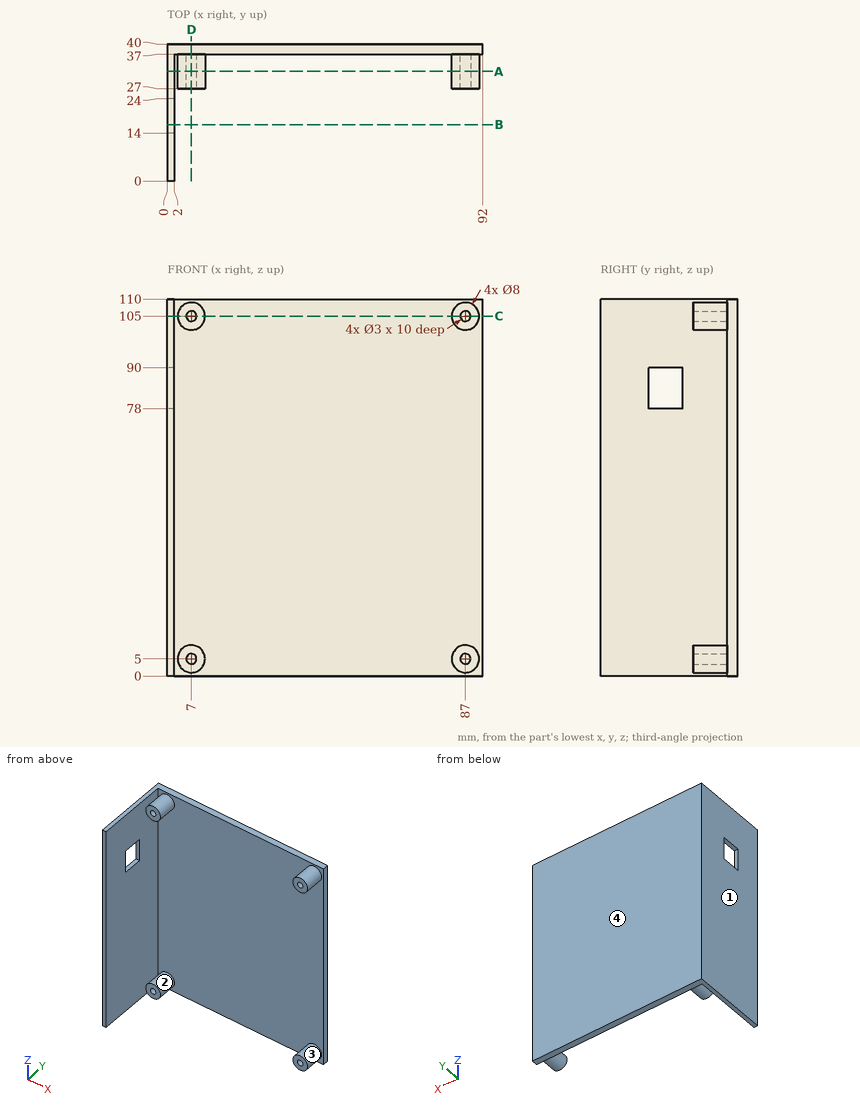
The figure shows three views and two pictorial views of one solid part (mm, origin at its lowest corner). Answer the questions. A direction names the side the tool comes from. Coordinates: 2 decimals unless noted, no trailing zeros. Loops run counter-clockwise (first coordinate to the right, second up) from the corner with the lowest first, then second, coordinate; pieces in that order, holes last.
(1) The mould has two halves that part along Z. Classify the marked faces 1 and 2: released by +Z, released by -Z, zero draft, split by the parting line, or undercut.
Solution:
face 1: zero draft
face 2: undercut
(2) Flat-ended cylindrical pins translate along their axes: pin 1 Ø2.5 at (x, z) = (6.5, 5.5) entering from -Y; pin 2 Ø1.5 at (x, z) = (86.5, 105.5) entering from -Y; pin 3 Ø6 at (y, z) = (15, 42.5) entering from -X; pin 4 Ø10 at (y, z) = (6, 44.5) entering from +X. Find the tip coordinate at first contact, or state that the pin passes through.
Solution:
pin 1: stops at y = 27
pin 2: stops at y = 37
pin 3: stops at x = 0
pin 4: stops at x = 2
(3) The part is cut by section B-B (y = 16.5). Determine the outline of the cut face in (x, z), and give its area (3 significant figures).
Solution:
outline: (0, 0) - (2, 0) - (2, 78) - (0, 78) - close; (0, 90) - (2, 90) - (2, 110) - (0, 110) - close
area: 196 mm2
(4) A tool of negligible diameter and unlimited length cuts with its end or side. For the marked faces 3 and 4, from which of +Z, -Z, +X, -X, +Y, -Y can it reach the whole face along a straight path? Write none if from no direction.
Solution:
face 3: -Y
face 4: +Z, -Z, +X, -X, +Y
(5) The part is cut by section D-D (x = 7). Determine the outline of the cut face in (y, z), and give its area (3 significant figures).
Solution:
outline: (27, 1) - (37, 1) - (37, 0) - (40, 0) - (40, 110) - (37, 110) - (37, 109) - (27, 109) - (27, 106.5) - (37, 106.5) - (37, 103.5) - (27, 103.5) - (27, 101) - (37, 101) - (37, 9) - (27, 9) - (27, 6.5) - (37, 6.5) - (37, 3.5) - (27, 3.5) - close
area: 430 mm2
(6) The part is cut by section C-C (z = 105). Determine the outline of the cut face in (x, y), and give its area (3 significant figures).
Solution:
outline: (0, 0) - (2, 0) - (2, 37) - (3, 37) - (3, 27) - (5.5, 27) - (5.5, 37) - (8.5, 37) - (8.5, 27) - (11, 27) - (11, 37) - (83, 37) - (83, 27) - (85.5, 27) - (85.5, 37) - (88.5, 37) - (88.5, 27) - (91, 27) - (91, 37) - (92, 37) - (92, 40) - (0, 40) - close
area: 450 mm2
(7) Consider line 1 along Z through (x, y) = (87, 30.25); line 2 along Y through (x, z) = (16, 83); line 3 along X through (y, z) = (2, 54). Determine where each line is inside the solid, lowest interval first.
Solution:
line 1: z = 1 to 3.5, 6.5 to 9, 101 to 103.5, 106.5 to 109
line 2: y = 37 to 40
line 3: x = 0 to 2
(8) The part is cut by section A-A (y = 32). Count the separate pieces of the cut face and the enclosed holes in it, and give its area (3 significant figures).
Solution:
separate pieces: 5
enclosed holes: 4
area: 393 mm2
